For this review, take the finished solid that the model builds, in its own axes (mm). A direction names the side the tool comes from. Round coordinates to 2 decimals unless told otherwise and drop trailing zeros. Order: outer loops, then holes, each group sorted by start corner. A loop starts at its lowest first (then second) coordinate and runs counter-clockwise, first axis right, second up. Notation, with made-up numbers: (69.5, 76.25) -> (82.5, 76.25) arc R36 cw to (82.5, 112.25) -> close; hole circle Ø11 at (29, 0.5). An arc over 180 degrees is marked (long way). Use a Markdown table: item, result. Add a question column.
1) Consider section B-B (y = 12). State the section outline as (x, z) points.
2) Machinability: for faces 4 (the face through (0, 0, 55)), 5 (the face through (16, -11, 14)), 6 (the face through (0.35, -36.346, 23.274)), which of the approach directions +Z, -Z, +X, -X, +Y, -Y give a long, thin tool a straight path to every point of the face, cutting with its end or side? Answer none if there is none.
3) Consider section A-A (y = -12). State the section outline as (x, z) points, plus the area to 3 significant figures.
4) Draft analysis for pull direction X (two halves, no side actions). For faces 1 (the face through (25, -3, 24)), 2 (the face through (0, 25, 27)), 3 (the face through (-16, -11, 14)), state which applies: pulls with the +X half, pulls with the -X half, needs draft (parallel to the pull), parting line crosses it, or undercut.
5) Wall thickness on line 1 along X through (y, z) = (-32, 55); line 2 along X through (y, z) = (-3.5, -20); line 3 along Y through (x, z) = (-2, 58.5): over which ranges is each line inside the solid? List them lowest first. Write a range as [from, to].
6) Consider section C-C (y = -45). State the section outline as (x, z) points.
7) Consider section D-D (y = 34). State the section outline as (x, z) points.
8) Clearance check with flat-ended pins moving along their axes: P1, Ø1.5, axis at x = 15.5, y = 0, coming from the +Z side; P2, Ø3, axis at x = 17, y = 23, coming from the +Z side; P3, Ø15, axis at x = -10, z = 14.5, coming from the +Y side. State where each tip first meets the part, or that it passes through.
```python
from build123d import *

# Parameters (mm, degrees)
EXTRUDE_8_DEPTH     = 25
EXTRUDE_START       = -25
SKETCH_12_R         = 25
EXTRUDE_9_DEPTH     = 80
FILLET_1_R          = 5
SKETCH_13_R         = 15
CUT_EXTRUDE_1_DEPTH = 80
SKETCH_14_R         = 25
EXTRUDE_10_DEPTH    = 25
CHAMFER_1_SIZE      = 3
SKETCH_15_R         = 15
CUT_EXTRUDE_2_DEPTH = 55
SKETCH_16_W         = 51.322430614
SKETCH_16_H         = 72.336093734
CUT_EXTRUDE_3_DEPTH = 16


with BuildPart() as part:
    # 草图10 → 凸台-拉伸8 (new, symmetric)
    with BuildSketch(Plane(origin=(0, 0, 0), x_dir=(0, 0, -1), z_dir=(1, 0, 0))):
        with BuildLine():
            Line((0, 25), (-55, 25))
            Line((-55, 25), (-55, -49.143520922))
            Line((-55, -49.143520922), (9.352376308, -23.184759162))
            ThreePointArc((9.352376308, -23.184759162), (24.541994408, 4.763455728), (0, 25))
        make_face()
    extrude(amount=EXTRUDE_8_DEPTH, both=True)

    # 草图12 → 凸台-拉伸9 (add)
    with BuildSketch(Plane(origin=(0, 25, 0), x_dir=(1, 0, 0), z_dir=(0, 1, 0)).offset(EXTRUDE_START)):
        with Locations(Location((0, -55, 0), (0, 0, 270))):
            Circle(SKETCH_12_R)
    extrude(amount=-EXTRUDE_9_DEPTH)

    # 圆角1
    fillet_1_edges = [part.edges().sort_by_distance(p)[0] for p in [
        (0, -80, 30),
    ]]
    fillet(fillet_1_edges, radius=FILLET_1_R)

    # 草图13 → 切除-拉伸1 (cut)
    with BuildSketch(Plane.XZ.offset(80)):
        with Locations(Location((0, 55, 0), (0, 0, 270))):
            Circle(SKETCH_13_R)
    extrude(amount=-CUT_EXTRUDE_1_DEPTH, mode=Mode.SUBTRACT)

    # 草图14 → 凸台-拉伸10 (add, symmetric)
    with BuildSketch(Plane(origin=(0, 25, 0), x_dir=(1, 0, 0), z_dir=(0, 1, 0))):
        with Locations(Location((0, -55, 0), (0, 0, 270))):
            Circle(SKETCH_14_R)
    extrude(amount=EXTRUDE_10_DEPTH, both=True)

    # 倒角1
    chamfer_1_edges = [part.edges().sort_by_distance(p)[0] for p in [
        (0, 50, 30),
    ]]
    chamfer(chamfer_1_edges, length=CHAMFER_1_SIZE)

    # 草图15 → 切除-拉伸2 (cut)
    with BuildSketch(Plane(origin=(25, 0, 0), x_dir=(0, 0, -1), z_dir=(1, 0, 0))):
        Circle(SKETCH_15_R)
    extrude(amount=-CUT_EXTRUDE_2_DEPTH, mode=Mode.SUBTRACT)

    # 草图16 → 切除-拉伸3 (cut, symmetric)
    with BuildSketch(Plane(origin=(0, 0, 0), x_dir=(0, 0, -1), z_dir=(1, 0, 0))):
        with Locations((4.773637783, -2.635053382)):
            Rectangle(SKETCH_16_W, SKETCH_16_H)
    extrude(amount=CUT_EXTRUDE_3_DEPTH, both=True, mode=Mode.SUBTRACT)


solid = part.part
```
Results list:
| question | item | result |
|---|---|---|
| 1 | outline | (-25, -21.93) -> (-16, -21.93) -> (-16, -9) -> (-25, -9) -> close; (-25, 9) -> (-16, 9) -> (-16, 20.89) -> (16, 20.89) -> (16, 9) -> (25, 9) -> (25, 55) arc R25 ccw to (-25, 55) -> close; (16, -21.93) -> (25, -21.93) -> (25, -9) -> (16, -9) -> close |
| 2 | face 4 | -Y |
| 2 | face 5 | -Z, +Y, -Y |
| 2 | face 6 | -Z, -Y |
| 3 | outline | (-25, -21.93) -> (-16, -21.93) -> (-16, -9) -> (-25, -9) -> close; (-25, 9) -> (-16, 9) -> (-16, 20.89) -> (16, 20.89) -> (16, 9) -> (25, 9) -> (25, 55) arc R25 ccw to (-25, 55) -> close; (16, -21.93) -> (25, -21.93) -> (25, -9) -> (16, -9) -> close; hole circle Ø30 at (0, 55) |
| 3 | area | 2,430 mm2 |
| 4 | face 1 | pulls with the +X half |
| 4 | face 2 | needs draft |
| 4 | face 3 | undercut |
| 5 | line 1 | [-25, -15], [15, 25] |
| 5 | line 2 | [-25, -16], [16, 25] |
| 5 | line 3 | [0, 50] |
| 6 | outline | (-25, 44.73) -> (-22.79, 44.73) arc R25 ccw to (22.79, 44.73) -> (25, 44.73) -> (25, 55) arc R25 ccw to (-25, 55) -> close; hole circle Ø30 at (0, 55) |
| 7 | outline | circle Ø50 at (0, 55) |
| 8 | P1 | z = 75.19 |
| 8 | P2 | z = 74.62 |
| 8 | P3 | y = 25 |
